```python
from build123d import *

# Parameters (mm, degrees)
SKETCH1_R           = 2.5
BOSS_EXTRUDE1_DEPTH = 24
SKETCH2_R           = 7.5
BOSS_EXTRUDE2_DEPTH = 2
FILLET1_R           = 1


with BuildPart() as part:
    # Sketch1 → Boss-Extrude1 (new body)
    with BuildSketch(Plane(origin=(0, 0, 0), x_dir=(1, 0, 0), z_dir=(0, 1, 0))):
        with Locations(Location((0, 0, 0), (0, 0, 270))):
            Circle(SKETCH1_R)
    extrude(amount=BOSS_EXTRUDE1_DEPTH)

    # Sketch2 → Boss-Extrude2 (add)
    with BuildSketch(Plane(origin=(0, 24, 0), x_dir=(1, 0, 0), z_dir=(0, 1, 0))):
        with Locations(Location((0, 0, 0), (0, 0, 270))):
            Circle(SKETCH2_R)
    extrude(amount=BOSS_EXTRUDE2_DEPTH)

    # Fillet1
    fillet1_edges = [part.edges().sort_by_distance(p)[0] for p in [
        (0, 24, -7.5),
        (0, 26, -7.5),
    ]]
    fillet(fillet1_edges, radius=FILLET1_R - 0.0001)  # a hair under: the kernel refuses the full size

    # Mirror1: part across plane


with BuildPart() as part_1:
    add(part.part)
    add(part.part.mirror(Plane.ZX))


solid = part_1.part
```
Could you check a few things on this model? Use its own coordinates, in mm. Round coordinates to 2 decimals unless told otherwise and drop trailing zeros. Loops run counter-clockwise (first coordinate to the right, second up) from the corner with the lowest first, then second, coordinate; pieces in that order, holes last.
Q1. For P1, Ø8, axis at y = 12.5, z = -4, coming from the -X side; P2, Ø1, axis at y = -9.5, z = 4.5, coming from the +X side, each with a flat end and sliding along its axis, tell me the tip position at first contact or that it passes through.
Q2. I want a section at C-C (y = 15.5). Write out the boundary of the cut face in (x, z), and give its area (3 significant figures).
Q3. Thinking about a two-plate mould opening in Y: for faces 1 (the flat face through (0, 26, 0)), 2 (the flat face through (0, 24, 3)), 3 (the cylindrical face through (-2.44, 0.34, -0.54)), 4 (the flat face through (0, -26, 0)), which applies, pulls with the +Y half, pulls with the -Y half, needs draft (parallel to the pull), parting line crosses it, or undercut?
Q4. Please list where these lines run through material, in increasing order: L1, parallel to Y at x = -4.25, z = -3.25; L2, parallel to X at y = 21, z = 0; L3, parallel to X at y = -1, z = 0.75.
Answer below:
1. P1: stops at x = -2.5
1. P2: passes through
2. outline: circle Ø5 at (0, 0)
2. area: 19.6 mm2
3. face 1: pulls with the +Y half
3. face 2: undercut
3. face 3: undercut
3. face 4: pulls with the -Y half
4. L1: y = -26 to -24, 24 to 26
4. L2: x = -2.5 to 2.5
4. L3: x = -2.38 to 2.38
